Print and shaded views of the part. All mm, measured from the part's lowest x, y and z. A direction names the side the tool comes from. Round coordinates to 2 decimals unless told otherwise and drop trailing zeros. Loops run counter-clockwise (first coordinate to the right, second up) from the corner with the lowest first, then second, coordinate; pieces in that order, holes last. Notation, with made-up numbers: (25, 66.25) - (54, 66.25) arc R16 ccw to (54, 80.25) - close; hole circle Ø7 at (1, 19.5). An arc over 180 degrees is marked (long way). Use one line per item in the form item = value.
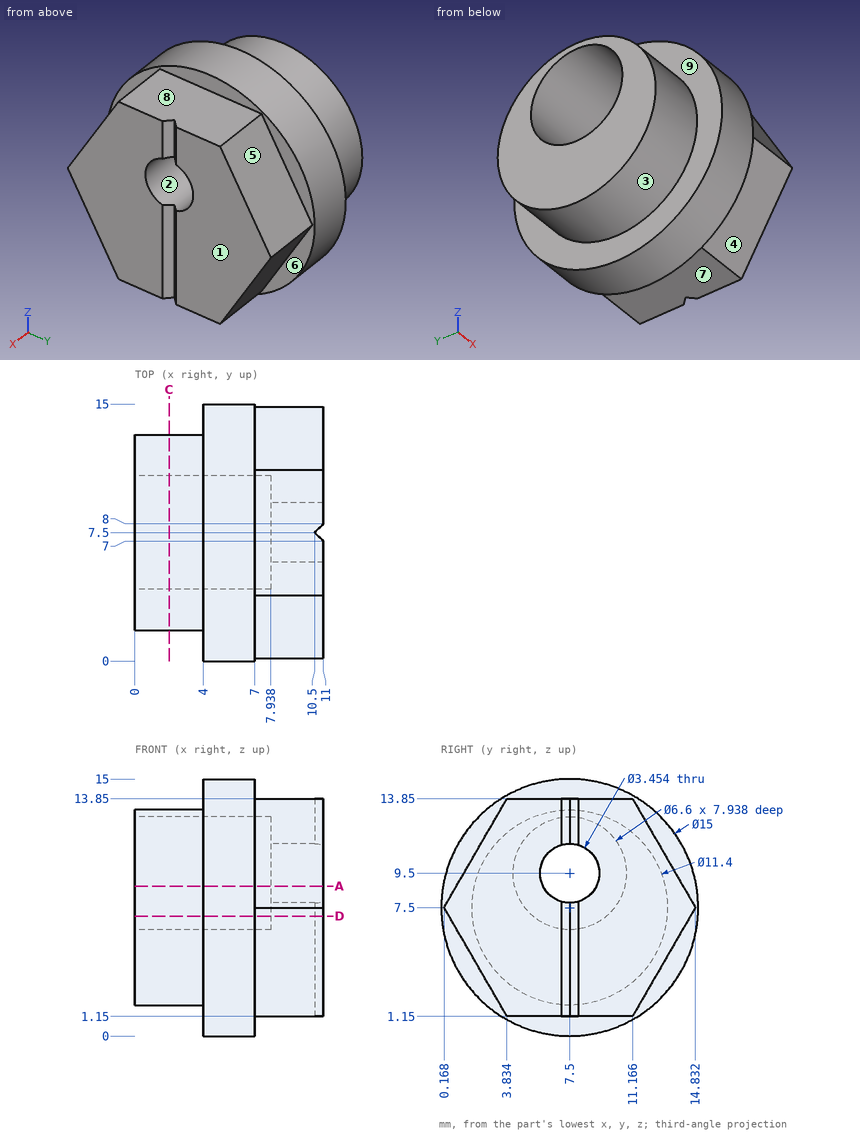
1) Drill centre lines: probe 1 along Z at (x, y) = (9.05, 7.5); probe 2 along X at (y, z) = (5, 13); probe 3 along Y at (x, z) = (5.25, 9.5). Where is each one in solid material? Low to high.
Report:
probe_1 = 1.15 to 7.77, 11.23 to 13.85
probe_2 = 4 to 11
probe_3 = 0.27 to 4.2, 10.8 to 14.73
2) Tool access for the marked faces 5, 6, 7, 8 and 9: list every direction of +Z, -Z, +X, -X, +Y, -Y with a clear straight run to the whole face (end or side of a thin tool).
Report:
face_5 = +Z, +X, +Y
face_6 = +X
face_7 = -Z, +X, +Y, -Y
face_8 = +Z, +X, +Y, -Y
face_9 = -X
3) Slice it at D-D (z = 7). Write the cut outline in (x, y) (1 decimal), plus the area to 3 significant figures.
Report:
outline = (0, 1.8) - (4, 1.8) - (4, 0) - (7, 0) - (7, 0.5) - (11, 0.5) - (11, 7) - (10.5, 7.5) - (11, 8) - (11, 14.5) - (7, 14.5) - (7, 15) - (4, 15) - (4, 13.2) - (0, 13.2) - (0, 9.7) - (7.9, 9.7) - (7.9, 5.3) - (0, 5.3) - close
area = 112 mm^2
4) Slice it at A-A (z = 8.75). Write the cut outline in (x, y) (1 decimal).
Report:
outline = (0, 1.9) - (4, 1.9) - (4, 0.1) - (7, 0.1) - (7, 0.9) - (11, 0.9) - (11, 5.9) - (7.9, 5.9) - (7.9, 4.3) - (0, 4.3) - close; (0, 10.7) - (7.9, 10.7) - (7.9, 9.1) - (11, 9.1) - (11, 14.1) - (7, 14.1) - (7, 14.9) - (4, 14.9) - (4, 13.1) - (0, 13.1) - close
5) Two-plate mould, pull along Y, no slides. Class the marked faces 1, 2, 3 and 4: +Y half, -Y half, draft (parallel to the pull), parting line (faces both ways), or undercut.
Report:
face_1 = draft
face_2 = undercut
face_3 = parting line
face_4 = -Y half
6) Flat gauge pins, fed straight in: pin 1 (4 mm diameter, centred on x = 8, y = 4, fed in from -Z); pin 2 (1 mm diameter, centred on x = 4, y = 11, fed in from +Z) (1 decimal); pin 3 (1.5 mm diameter, centred on x = 9.5, z = 10, fed in from +Y). Where does each tip first touch, or does it go through?
Report:
pin_1 = 0.21
pin_2 = 14.4
pin_3 = 13.82
7) Slice it at C-C (x = 2). Write the cut outline in (y, z).
Report:
outline = circle Ø11.4 at (7.5, 7.5); hole circle Ø6.6 at (7.5, 9.5)
